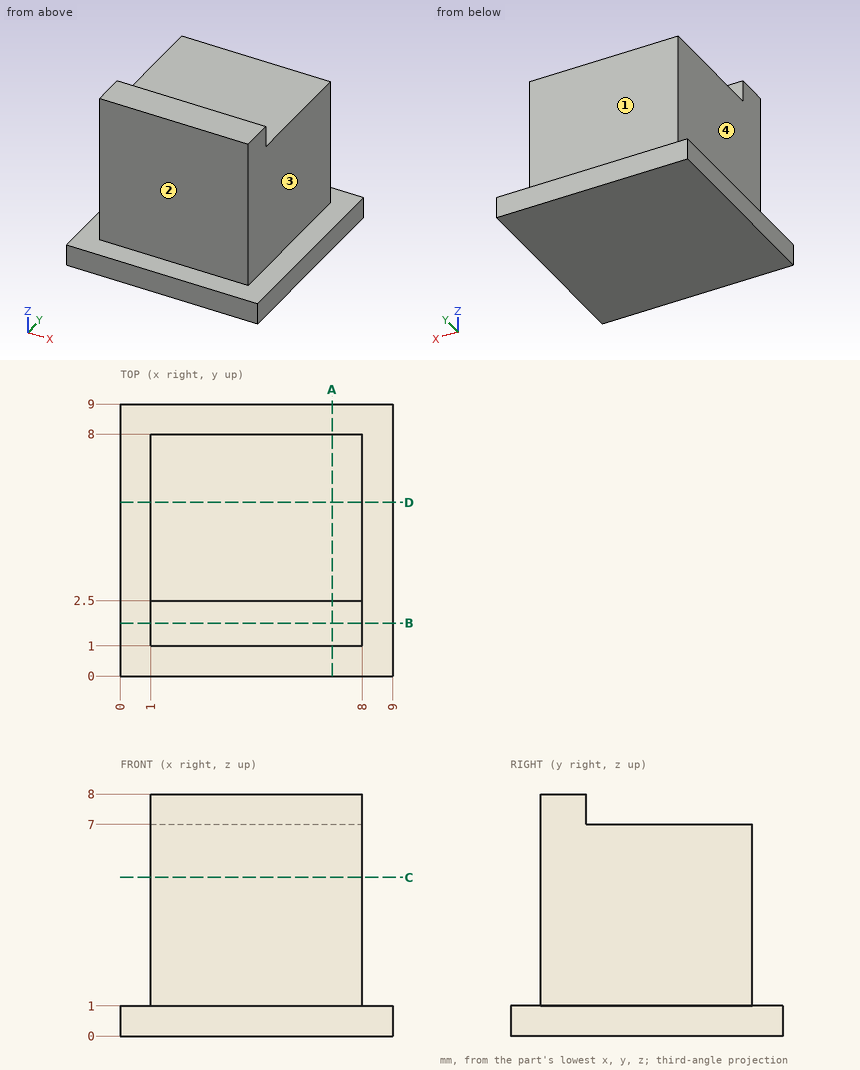
Could you check a few things on this drawing? It's one solid part, dimensions in mm from its lowest x, y, z. A direction names the side the tool comes from. Coordinates: 2 decimals unless noted, no trailing zeros. Order: outer loops, then holes, each group sorted by start corner. A loop starts at its lowest first (then second) coordinate and runs counter-clockwise, first axis right, second up. Notation, with made-up numbers: M 87.25,88.5 L 97.25,88.5 A22 ccw 97.25,110.5 Z; hole C 73.25,-12 d10. An arc over 180 degrees is marked long. Use one line per item in the form item = value. Start each with the question number.
1. Suppose I cut it at A-A on x = 7. Write out the boundary of the cut face in (y, z).
2. Suppose I cut it at B-B on y = 1.75. Write out the boundary of the cut face in (x, z).
3. Please list where these lines run through material, in increasing order: line 1 (Z direction, x = 5.5, y = 8.5); line 2 (Y direction, x = 5, z = 5.75).
4. On a 3-axis mill with a long thin cutter (end or side, diameter ignored), from which of +Z, -Z, +X, -X, +Y, -Y can I reach the whole of each face in a straight line? I mean the marked faces 1, 2, 3 and 4. Say none if no direction works.
5. Suppose I cut it at D-D on y = 5.75. Write out the boundary of the cut face in (x, z).
6. For pin 1 (2.5 mm diameter, centred on x = 3, y = 5.5, fed in from +Z); pin 2 (2 mm diameter, centred on y = 4, z = 4.5, fed in from -X); pin 3 (3 mm diameter, centred on y = 3, z = 3.5, fed in from +X); pin 4 (5 mm diameter, centred on x = 5.5, y = 2, fed in from -Z), each with a flat end and sliding along its axis, tell me the tip position at first contact or that it passes through.
7. Suppose I cut it at C-C on z = 5.25. Write out the boundary of the cut face in (x, y), then the cut area to 3 significant figures.
Geometry says:
q1.outline = M 0,0 L 9,0 L 9,1 L 8,1 L 8,7 L 2.5,7 L 2.5,8 L 1,8 L 1,1 L 0,1 Z
q2.outline = M 0,0 L 9,0 L 9,1 L 8,1 L 8,8 L 1,8 L 1,1 L 0,1 Z
q3.line_1 = 0 to 1
q3.line_2 = 1 to 8
q4.face_1 = +Z, +X, -X, +Y
q4.face_2 = +Z, +X, -X, -Y
q4.face_3 = +Z, +X, +Y, -Y
q4.face_4 = +Z, -X, +Y, -Y
q5.outline = M 0,0 L 9,0 L 9,1 L 8,1 L 8,7 L 1,7 L 1,1 L 0,1 Z
q6.pin_1 = 7
q6.pin_2 = 1
q6.pin_3 = 8
q6.pin_4 = 0
q7.outline = M 1,1 L 8,1 L 8,8 L 1,8 Z
q7.area = 49.0 mm^2
